Study the drawing (mm; zero at the part's minimum x, y, z) and answer. A direction names the side the tool comes from. Round coordinates to 2 decimals unless told otherwise and drop trailing zeros. Loops run counter-clockwise (first coordinate to the right, second up) from the corner with the lowest first, then second, coordinate; pieces in that order, holes last. Notation, with made-up numbers: (39.5, 12.5) -> (94.5, 12.5) arc R29 cw to (94.5, 46.5) -> close; hole circle Ø7 at (27, -19.5). An arc over 180 degrees is marked (long way). Use one line per item in the form item = value.
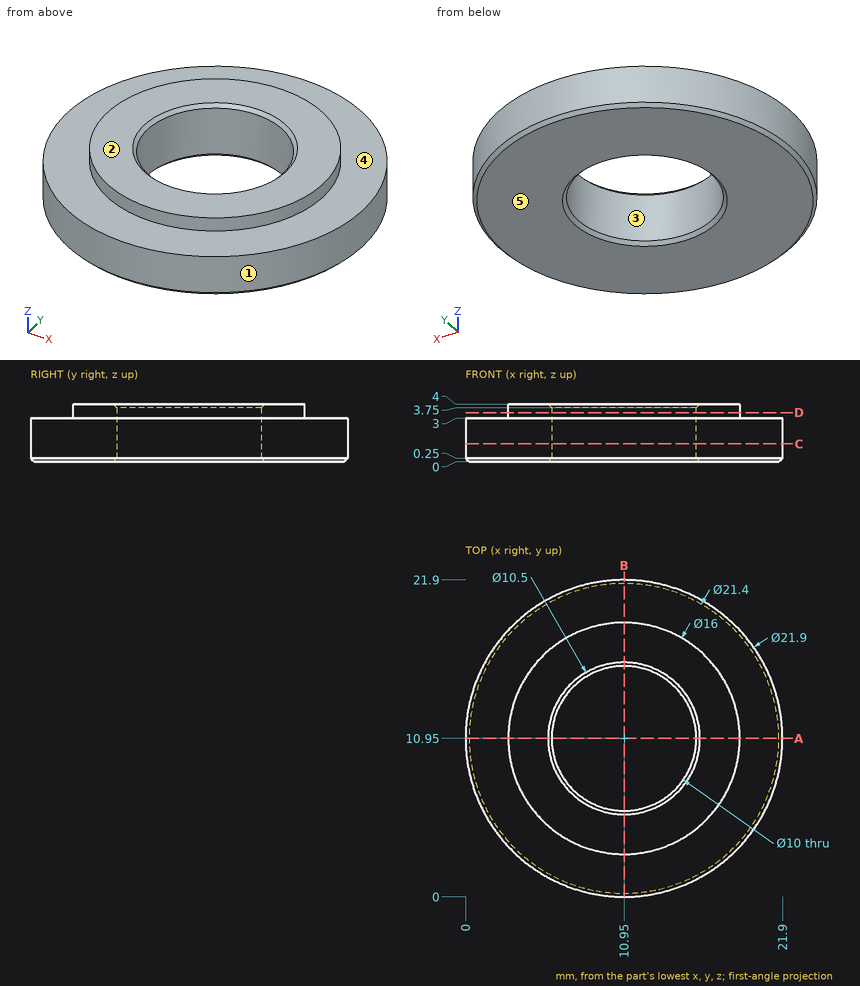
(1) Find section C-C, the plane z = 1.25. Write down the section's boundary in (x, y).
Completed:
outline = circle Ø21.9 at (10.95, 10.95); hole circle Ø10 at (10.95, 10.95)
(2) Find section A-A, the plane y = 10.95. Write down the section's boundary in (x, z).
Completed:
outline = (0, 0.25) -> (0.25, 0) -> (5.7, 0) -> (5.95, 0.25) -> (5.95, 3.75) -> (5.7, 4) -> (2.95, 4) -> (2.95, 3) -> (0, 3) -> close; (15.95, 0.25) -> (16.2, 0) -> (21.65, 0) -> (21.9, 0.25) -> (21.9, 3) -> (18.95, 3) -> (18.95, 4) -> (16.2, 4) -> (15.95, 3.75) -> close
(3) For a pull along Y with two mould halves and no side action, classify the marked faces 1, 2 and 3 as +Y half, -Y half, draft (parallel to the pull), parting line (faces both ways), or undercut.
Completed:
face_1 = parting line
face_2 = draft
face_3 = undercut
(4) Find section D-D, the plane z = 3.4. Write down the section's boundary in (x, y), then the cut area to 3 significant figures.
Completed:
outline = circle Ø16 at (10.95, 10.95); hole circle Ø10 at (10.95, 10.95)
area = 123 mm2
(5) For the marked faces 4 and 5, determine the directions among +Z, -Z, +X, -X, +Y, -Y from which every point of the face is accessible in a straight line to the end or side of a thin tool.
Completed:
face_4 = +Z
face_5 = -Z, +X, -X, +Y, -Y
(6) Consider L1, parallel to Y at x = 10.95, z = 2.85; L2, parallel to Z at x = 3, y = 14.5; L3, parallel to X at y = 14.25, z = 3.25. Determine where each line is inside the solid, lowest interval first.
Completed:
L1 = 0 to 5.95, 15.95 to 21.9
L2 = 0 to 3
L3 = 3.66 to 7.19, 14.71 to 18.24
(7) Given P1, Ø12, axis at x = 6, y = 6, coming from the -Z side; P2, Ø1.5, axis at x = 17.5, z = 3, coming from the +Y side; P3, Ø1.5, axis at x = 4, z = 2.5, coming from the +Y side; P4, Ø1.5, axis at y = 17.5, z = 2, coming from the +X side, each flat-ended and moving along its own axis, determine where each tip first touches the part or whether it passes through.
Completed:
P1 = 0
P2 = 20.24
P3 = 19.98
P4 = 20.24
